Can you work these out from the model? Positions are in its coordinate system, mm. Face numbers are marked on the shaded views. A direction names the side the tool comes from. Give positions to 0.01 mm unless a question says otherwise; leave off trailing zeros. Order: outer loops, then holes, each group sorted by start corner. A loop starts at its lowest first (then second) coordinate and runs counter-clockwise, first axis right, second up. Notation, with made-up numbers: (-15, 48) -> (-2, 48) arc R20 cw to (-2, 86) -> close; hole circle Ø10 at (-3.5, 4.5). An arc over 180 degrees is marked (long way). Answer as a JSON object with one key per item and string values.
Autodesk Inventor part; units mm, degrees
ref_plane "YZ Plane" through (0, 0, 0) normal (1, 0, 0) x (0, 1, 0)
ref_plane "XZ Plane" through (0, 0, 0) normal (0, 1, 0) x (-1, 0, 0)
ref_plane "XY Plane" through (0, 0, 0) normal (0, 0, 1) x (1, 0, 0)
sketch "Sketch1" plane through (0, 0, 0) normal (0, 0, 1) x (1, 0, 0)
  circle A0 centre (0, 0) radius 6.5
  dimension "d0" = 13
extrude "Extrusion1" add sketch "Sketch1" along normal blind 30
sketch "Sketch3" plane through (0, 0, 30) normal (0, 0, 1) x (1, 0, 0)
  circle A0 centre (0, 0) radius 90
  dimension "d3" = 180
sketch "Sketch4" plane through (0, 0, 0) normal (0, 0, -1) x (-1, 0, 0)
  circle A0 centre (0, 0) radius 2
  dimension "d4" = 4
extrude "Extrusion2" cut sketch "Sketch4" against normal blind 20
ref_plane "Work Plane2" through (0.2663, 6.4945, 0) normal (0.041, 0.9992, 0) x (-0.9992, 0.041, 0)
ref_plane "Work Plane1" through (-27.6829, 45.9903, 12) normal (0.041, 0.9992, 0) x (-0.9992, 0.041, 0)
ref_plane "Work Plane4" through (0.2663, 6.4945, 0) normal (0.041, 0.9992, 0) x (-0.9992, 0.041, 0)
ref_plane "Work Plane3" through (19.1559, -19.777, -43.8) normal (0.041, 0.9992, 0) x (-0.9992, 0.041, 0)
sketch "Sketch5" plane through (0.2663, 6.4945, 0) normal (0.041, 0.9992, 0) x (-0.9992, 0.041, 0)
  line L0 (0, 0) -> (0, 20)
  line L1 (0, 20) -> (0, 5)
  line L2 (0, 5) -> (0, 10)
  circle A0 centre (0, 10) radius 1.2
  circle A1 centre (0, 5) radius 1.2
  dimension "d7" = 20
  dimension "d8" = 15
  dimension "d9" = 5
  dimension "d10" = 2.4
extrude "Extrusion3" cut sketch "Sketch5" against normal blind 20
sketch "Sketch6" plane through (0, 0, 30) normal (0, 0, 1) x (1, 0, 0)
  circle A0 centre (0, 0) radius 90
  dimension "d13" = 180
extrude "Extrusion4" add sketch "Sketch6" along normal blind 5
properties part number "plošča za vrtenje"
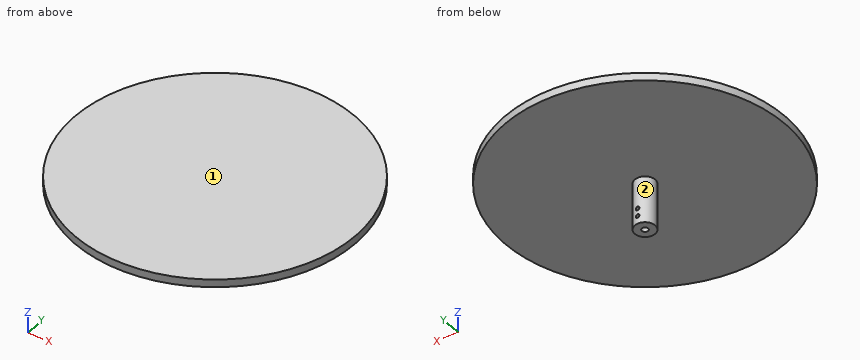
1. If we section it at B-B on x = 30.5: Please give me the cut outline in (y, z), then the cut area to 3 significant figures.
Worked answers:
{"outline": "(-84.67, 30) -> (84.67, 30) -> (84.67, 35) -> (-84.67, 35) -> close", "area": "847 mm²"}
2. If we section it at A-A on z = 17.5: Please give me the cut outline in (x, y), then the cut area to 3 significant figures.
Worked answers:
{"outline": "circle Ø13 at (0, 0); hole circle Ø4 at (0, 0)", "area": "120 mm²"}
3. Will these pins go through, and if not, where does the flat tip stop? pin 1 Ø10 at (x, y) = (21.5, 30) entering from -Z; pin 2 Ø12 at (y, z) = (-34.5, 24.5) entering from +X; pin 3 Ø12 at (y, z) = (-43.5, 31) entering from -X.
Worked answers:
{"pin 1": "z = 30", "pin 2": "x = 84.08", "pin 3": "x = -81.82"}
4. If we section it at C-C on y = -13.5: Please give me the cut outline in (x, z).
Worked answers:
{"outline": "(-88.98, 30) -> (88.98, 30) -> (88.98, 35) -> (-88.98, 35) -> close"}
5. Please list where these lines run through material, in increasing order: L1, parallel to Y at x = 0, z = 15; L2, parallel to Z at x = 5.5, y = -18; L3, parallel to X at y = 35.5, z = 33.
Worked answers:
{"L1": "-6.5 to -2, 2 to 6.5", "L2": "30 to 35", "L3": "-82.7 to 82.7"}
6. For the marked faces 1 and 2, which set-ups out of +Z, -Z, +X, -X, +Y, -Y let a thin tool reach every point of the face, with its end or its side?
Worked answers:
{"face 1": "+Z, +X, -X, +Y, -Y", "face 2": "-Z"}
